Can you work these out from the drawing? Everything is in mm from the part's minimum corner. Give positions to 0.01 mm unless a question says otherwise; leave off trailing zeros. Write each loop counter-clockwise with the first axis right and the second up, starting at its lowest first coordinate (ties: lowest second). Pieces come first, ordered by that corner, then holes. Notation, with made-up numbers: (61.25, 43) - (113.25, 43) arc R17 cw to (113.25, 59) - close; hole circle Ø11 at (10.5, 30). An arc over 180 degrees is marked (long way). Answer in a Markdown table with one row per item.
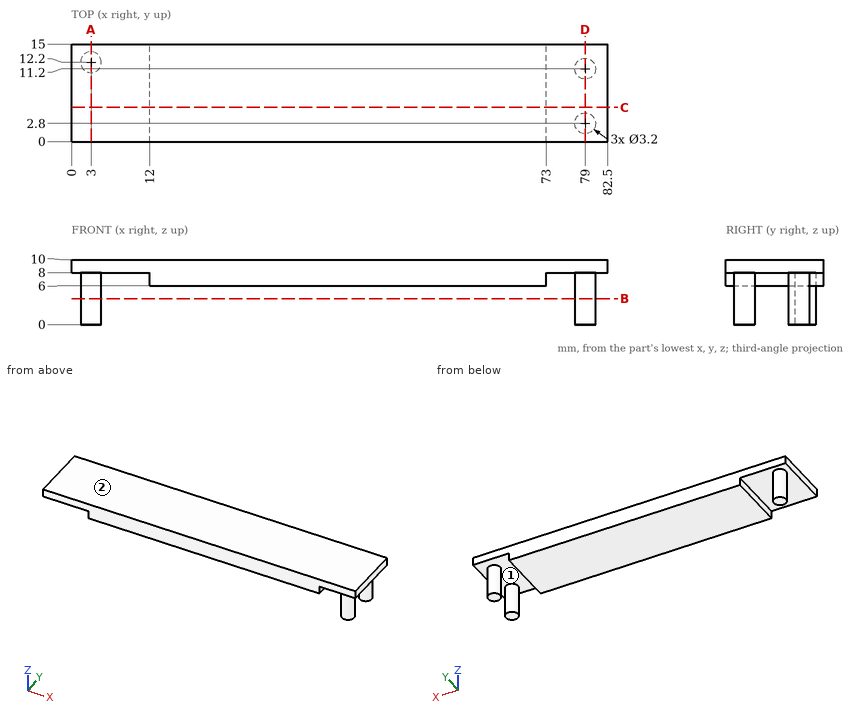
1) Imagine slicing it at A-A (x = 3). List the corners of the cut face in (y, z) for me, then the cut area to 3 significant figures.
Check values:
| item | result |
|---|---|
| outline | (0, 8) - (10.6, 8) - (10.6, 0) - (13.8, 0) - (13.8, 8) - (15, 8) - (15, 10) - (0, 10) - close |
| area | 55.6 mm2 |
2) Imagine slicing it at D-D (x = 79). List the corners of the cut face in (y, z) for me, then the cut area to 3 significant figures.
Check values:
| item | result |
|---|---|
| outline | (0, 8) - (1.2, 8) - (1.2, 0) - (4.4, 0) - (4.4, 8) - (9.6, 8) - (9.6, 0) - (12.8, 0) - (12.8, 8) - (15, 8) - (15, 10) - (0, 10) - close |
| area | 81.2 mm2 |
3) We'd pull the mould along X, two halves only. Please class the marked faces 1 and 2: +X half, -X half, draft (parallel to the pull), parting line (faces both ways), or undercut.
Check values:
| item | result |
|---|---|
| face 1 | undercut |
| face 2 | draft |
4) Imagine slicing it at C-C (y = 5.25). List the corners of the cut face in (x, z) for me, then the cut area to 3 significant figures.
Check values:
| item | result |
|---|---|
| outline | (0, 8) - (12, 8) - (12, 6) - (73, 6) - (73, 8) - (82.5, 8) - (82.5, 10) - (0, 10) - close |
| area | 287 mm2 |
5) If I drill on line 1 (Z direction, x = 63, y = 6); line 2 (X direction, y = 11.25, z = 4.5); line 3 (Z direction, x = 6, y = 6), over which ranges is the centre line in solid material (lowest first)?
Check values:
| item | result |
|---|---|
| line 1 | z = 6 to 10 |
| line 2 | x = 1.71 to 4.29, 77.4 to 80.6 |
| line 3 | z = 8 to 10 |
6) Imagine slicing it at B-B (z = 4). List the corners of the cut face in (x, y) for me.
Check values:
| item | result |
|---|---|
| outline | circle Ø3.2 at (3, 12.2); circle Ø3.2 at (79, 2.8); circle Ø3.2 at (79, 11.2) |
7) Will these pins go through, and if not, where does the flat tip stop? P1, Ø5, axis at x = 71.5, y = 2.5, coming from the -Z side; P2, Ø6, axis at x = 8.5, y = 5, coming from the -Z side.
Check values:
| item | result |
|---|---|
| P1 | stops at z = 6 |
| P2 | stops at z = 8 |
